Build history of the part. All positions in model axes, mm. A direction names the side the tool comes from. Give positions to 0.01 mm unless a question says otherwise; leave off trailing zeros. Loops run counter-clockwise (first coordinate to the right, second up) from the corner with the lowest first, then second, coordinate; pieces in that order, holes last. Notation, with made-up numbers: (3, -3) -> (7, -3) arc R17 cw to (7, 16) -> close; hole circle Ø3 at (9, -11.75). An arc over 180 degrees is marked (long way). Answer in a Markdown table with one row per item. Add a question column.
from build123d import *

# Parameters (mm, degrees)
F0_W     = 40
F0_H     = 145
F1_DEPTH = 75
F2_W     = 40
F2_H     = 50
F2_R     = 4
F3_DEPTH = 50
F4_R     = 4.542439
F4_R_2   = 4.801552
F5_DEPTH = 25


with BuildPart() as f1:
    # F0 (on Top) → F1 (new body)
    with BuildSketch(Plane.XY):
        Rectangle(F0_W, F0_H)
    extrude(amount=F1_DEPTH)

    # F2 (on face) → F3 (cut)
    with BuildSketch(Plane.XY.offset(75)):
        with Locations((0, -47.5)):
            Rectangle(F2_W, F2_H)
        with Locations((0, -62.5)):
            Circle(F2_R, mode=Mode.SUBTRACT)
        with Locations((0, 47.5)):
            Rectangle(F2_W, F2_H)
        with Locations((0, 62.5)):
            Circle(F2_R, mode=Mode.SUBTRACT)
    extrude(amount=-F3_DEPTH, mode=Mode.SUBTRACT)

    # F4 (on face) → F5 (cut)
    with BuildSketch(Plane.XY.offset(75)):
        with Locations((0, 62.5)):
            Circle(F4_R)
        with Locations((0, -62.5)):
            Circle(F4_R_2)
    extrude(amount=-F5_DEPTH, mode=Mode.SUBTRACT)


solid = f1.part
(1) Saw through at D-D, the plane z = 53. List the corners of the cut face in (x, y).
(2) 3-axis set-ups, long thin cutter, end or side, ignore diameter. For faces 1 (the cylindrical face through (-0.867, -66.405, 37.675)), 2 (the flat face through (0, 63, 50)), 3 (the flat face through (0, 0, 75)), 4 (the flat face through (0, 1, 0)), 5 (the flat face through (0, -62, 50)): which of +Z, -Z, +X, -X, +Y, -Y reach the whole face in a straight line?
(3) Wall check: line 1 along Y through (x, z) = (-3.5, 26); line 2 along Y through (x, z) = (-5.5, 46); line 3 along Z through (x, y) = (9, 60). Give the ranges that are in metal, low to high. Write a range as from..to.
(4) Saw through at C-C, the plane y = -62.5. List the corners of the cut face in (x, z), then the cut area to 3 significant figures.
(5) Saw through at B-B, the plane x = 0. List the corners of the cut face in (y, z).
(6) Saw through at A-A, the plane z = 29. List the corners of the cut face in (x, y), then the cut area to 3 significant figures.
(7) Flat gauge pins, fed straight in: pin 1 Ø20 at (x, z) = (-2.5, 38.5) entering from +Y; pin 2 Ø4 at (x, z) = (11.5, 42) entering from +Y; pin 3 Ø9 at (x, y) = (0, -61) entering from +Z. Where does each tip first touch, or does it go through?
(8) Two-plate mould, pull along Y, no slides. Class faces 6 (the cylindrical face through (-0.867, 58.595, 37.675)), 7 (the flat face through (0, -72.5, 12)), 8 (the flat face through (-20, -1, 29)): released by +Y, released by -Y, zero draft, split by the parting line, or undercut.
Worked answers:
| question | item | result |
|---|---|---|
| 1 | outline | (-20, -22.5) -> (20, -22.5) -> (20, 22.5) -> (-20, 22.5) -> close |
| 2 | face 1 | +Z |
| 2 | face 2 | +Z, +X, -X, +Y |
| 2 | face 3 | +Z, +X, -X, +Y, -Y |
| 2 | face 4 | -Z, +X, -X, +Y, -Y |
| 2 | face 5 | +Z, +X, -X, -Y |
| 3 | line 1 | -64.44..-60.56, -22.5..22.5, 60.56..64.44 |
| 3 | line 2 | -22.5..22.5 |
| 3 | line 3 | 0..25 |
| 4 | outline | (-20, 0) -> (20, 0) -> (20, 25) -> (4, 25) -> (4, 50) -> (-4, 50) -> (-4, 25) -> (-20, 25) -> close |
| 4 | area | 1,200 mm^2 |
| 5 | outline | (-72.5, 0) -> (72.5, 0) -> (72.5, 25) -> (66.5, 25) -> (66.5, 50) -> (58.5, 50) -> (58.5, 25) -> (22.5, 25) -> (22.5, 75) -> (-22.5, 75) -> (-22.5, 25) -> (-58.5, 25) -> (-58.5, 50) -> (-66.5, 50) -> (-66.5, 25) -> (-72.5, 25) -> close |
| 6 | outline | (-20, -22.5) -> (20, -22.5) -> (20, 22.5) -> (-20, 22.5) -> close; circle Ø8 at (0, -62.5); circle Ø8 at (0, 62.5) |
| 6 | area | 1,900 mm^2 |
| 7 | pin 1 | y = 66.5 |
| 7 | pin 2 | y = 22.5 |
| 7 | pin 3 | z = 50 |
| 8 | face 6 | undercut |
| 8 | face 7 | released by -Y |
| 8 | face 8 | zero draft |
